```python
from build123d import *

# Parameters (mm, degrees)
SKETCH_1_R          = 17.5
EXTRUDE_1_DEPTH     = 3.5
CUT_EXTRUDE_1_DEPTH = 2.5
FILLET_1_R          = 10
SKETCH_3_R          = 17.5
CUT_EXTRUDE_2_DEPTH = 2.5
FILLET_2_R          = 1
FILLET_3_R          = 1
SKETCH_4_R          = 1.4
SKETCH_4_R_2        = 1
SKETCH_4_R_3        = 1.5
SKETCH_4_R_4        = 5
CUT_EXTRUDE_3_DEPTH = 25.99499964


with BuildPart() as part:
    # ｽｹｯﾁ1 → ﾎﾞｽ - 押し出し1 (new body)
    with BuildSketch(Plane.XY):
        Circle(SKETCH_1_R)
    extrude(amount=EXTRUDE_1_DEPTH)

    # ｽｹｯﾁ2 → ｶｯﾄ - 押し出し1 (cut)
    with BuildSketch(Plane.XY.offset(3.5)):
        with BuildLine():
            ThreePointArc((-2.853095764, 12.580534351), (-11.171727709, 6.45), (-12.321610223, -3.819413764))
            ThreePointArc((-12.321610223, -3.819413764), (-13.856406461, -8), (-9.468514459, -8.761120587))
            ThreePointArc((-9.468514459, -8.761120587), (0, -12.9), (9.468514459, -8.761120587))
            ThreePointArc((9.468514459, -8.761120587), (13.856406461, -8), (12.321610223, -3.819413764))
            ThreePointArc((12.321610223, -3.819413764), (11.171727709, 6.45), (2.853095764, 12.580534351))
            ThreePointArc((2.853095764, 12.580534351), (0, 16), (-2.853095764, 12.580534351))
        make_face()
    extrude(amount=-CUT_EXTRUDE_1_DEPTH, mode=Mode.SUBTRACT)

    # ﾌｨﾚｯﾄ1
    fillet_1_edges = [part.edges().sort_by_distance(p)[0] for p in [
        (2.853095764, 12.580534351, 2.25),
        (12.321610223, -3.819413764, 2.25),
        (9.468514459, -8.761120587, 2.25),
        (-9.468514459, -8.761120587, 2.25),
        (-12.321610223, -3.819413764, 2.25),
        (-2.853095764, 12.580534351, 2.25),
    ]]
    fillet(fillet_1_edges, radius=FILLET_1_R)

    # ｽｹｯﾁ3 → ｶｯﾄ - 押し出し2 (cut)
    with BuildSketch(Plane(origin=(0, 0, 0), x_dir=(-1, 0, 0), z_dir=(0, 0, -1))):
        Circle(SKETCH_3_R)
        with BuildLine():
            ThreePointArc((11.580900059, -10.442854922), (14.722431864, -8.5), (14.834227681, -4.807926189))
            ThreePointArc((14.834227681, -4.807926189), (14.092365761, -2.7019505), (13.8917733, -0.478157484))
            ThreePointArc((13.8917733, -0.478157484), (12.037753113, 6.95), (6.531790122, 12.269707324))
            ThreePointArc((6.531790122, 12.269707324), (4.706225108, 13.555321998), (3.253327621, 15.250781111))
            ThreePointArc((3.253327621, 15.250781111), (0, 17), (-3.253327621, 15.250781111))
            ThreePointArc((-3.253327621, 15.250781111), (-4.706225108, 13.555321998), (-6.531790122, 12.269707324))
            ThreePointArc((-6.531790122, 12.269707324), (-12.037753113, 6.95), (-13.8917733, -0.478157484))
            ThreePointArc((-13.8917733, -0.478157484), (-14.092365761, -2.7019505), (-14.834227681, -4.807926189))
            ThreePointArc((-14.834227681, -4.807926189), (-14.722431864, -8.5), (-11.580900059, -10.442854922))
            ThreePointArc((-11.580900059, -10.442854922), (-9.386140653, -10.853371498), (-7.359983178, -11.791549839))
            ThreePointArc((-7.359983178, -11.791549839), (0, -13.9), (7.359983178, -11.791549839))
            ThreePointArc((7.359983178, -11.791549839), (9.386140653, -10.853371498), (11.580900059, -10.442854922))
        make_face(mode=Mode.SUBTRACT)
    extrude(amount=-CUT_EXTRUDE_2_DEPTH, mode=Mode.SUBTRACT)

    # ﾌｨﾚｯﾄ2
    fillet_2_edges = [part.edges().sort_by_distance(p)[0] for p in [
        (-13.856406461, -8, 3.5),
        (0, -12.9, 3.5),
        (-11.171727709, 6.45, 3.5),
        (0, 16, 3.5),
        (11.171727709, 6.45, 3.5),
        (13.856406461, -8, 3.5),
        (-4.033471592, 12.815455316, 3.5),
        (4.033471592, 12.815455316, 3.5),
        (13.115245661, -2.914638794, 3.5),
        (9.081774068, -9.900816522, 3.5),
        (-9.081774068, -9.900816522, 3.5),
        (-13.115245661, -2.914638794, 3.5),
    ]]
    fillet(fillet_2_edges, radius=FILLET_2_R)

    # ﾌｨﾚｯﾄ3
    fillet_3_edges = [part.edges().sort_by_distance(p)[0] for p in [
        (-9.386140653, -10.853371498, 0),
        (0, -13.9, 0),
        (9.386140653, -10.853371498, 0),
        (14.722431864, -8.5, 0),
        (14.092365761, -2.7019505, 0),
        (12.037753113, 6.95, 0),
        (4.706225108, 13.555321998, 0),
        (0, 17, 0),
        (-4.706225108, 13.555321998, 0),
        (-12.037753113, 6.95, 0),
        (-14.092365761, -2.7019505, 0),
        (-14.722431864, -8.5, 0),
    ]]
    fillet(fillet_3_edges, radius=FILLET_3_R)

    # ｽｹｯﾁ4 → ｶｯﾄ - 押し出し3 (cut, through all)
    with BuildSketch(Plane.XY.offset(3.5)):
        with Locations((0, 13.1)):
            Circle(SKETCH_4_R)
        with Locations((0, -15.5)):
            Circle(SKETCH_4_R_2)
        with Locations((11.34493279, -6.55)):
            Circle(SKETCH_4_R)
        with Locations((-13.423393759, 7.75)):
            Circle(SKETCH_4_R_2)
        with Locations((-11.34493279, -6.55)):
            Circle(SKETCH_4_R)
        with Locations((13.423393759, 7.75)):
            Circle(SKETCH_4_R_2)
        with Locations((0, 8)):
            Circle(SKETCH_4_R_3)
        Circle(SKETCH_4_R_4)
        with Locations((0, -8)):
            Circle(SKETCH_4_R_3)
    extrude(amount=-CUT_EXTRUDE_3_DEPTH, mode=Mode.SUBTRACT)


solid = part.part
```
Here's how the part is built. I have some questions about the finished solid (model axes, mm). A direction names the side the tool comes from. Give positions to 0.01 mm unless a question says otherwise; leave off trailing zeros. Put each result on its own line as item: value. Start each with the question number.
(1) Will these pins go through, and if not, where does the flat tip stop? pin 1 Ø1.8 at (x, y) = (0, -15.5) entering from +Z; pin 2 Ø3.5 at (x, y) = (11.34, -6.55) entering from +Z; pin 3 Ø2.5 at (x, y) = (-13.42, 7.75) entering from -Z.
(2) I want a section at A-A on x = 0. State how many separate pieces and enclosed holes the cut face has, then the cut area to 3 significant figures.
(3) If we mould it in two halves opening along X, with no side actions, what happens to faces 1 (the cylindrical face through (14.086, -2.671, 1.74)), 2 (the cylindrical face through (-13.876, -7.965, 1.76)), 3 (the cylindrical face through (-9.36, -10.86, 1.74))? For each: +X half, -X half, draft (parallel to the pull), parting line (faces both ways), or undercut.
(4) For faces 4 (the flat face through (8, -12, 2.5)), 5 (the cylindrical face through (-4.729, 13.534, 1.74)), 6 (the flat face through (3, -5, 1)), which set-ups out of +Z, -Z, +X, -X, +Y, -Y let a thin tool reach every point of the face, with its end or its side?
(5) I need wall thicknesses on line 1 along Z through (x, y) = (-10, 1.5); line 2 along Y through (x, z) = (-9, 2.25); line 3 along Z through (x, y) = (-6.5, 16). Which ranges of each line are inside material? Lowest first, please. Write a range as [from, to].
Answer block:
1. pin 1: through
1. pin 2: z = 1
1. pin 3: z = 2.5
2. separate pieces: 6
2. enclosed holes: 0
2. area: 18.3 mm^2
3. face 1: +X half
3. face 2: undercut
3. face 3: -X half
4. face 4: -Z
4. face 5: -Z, -X, +Y
4. face 6: +Z
5. line 1: [0, 1]
5. line 2: [-10.99, -9.93], [9.24, 10.59]
5. line 3: [2.5, 3.5]
